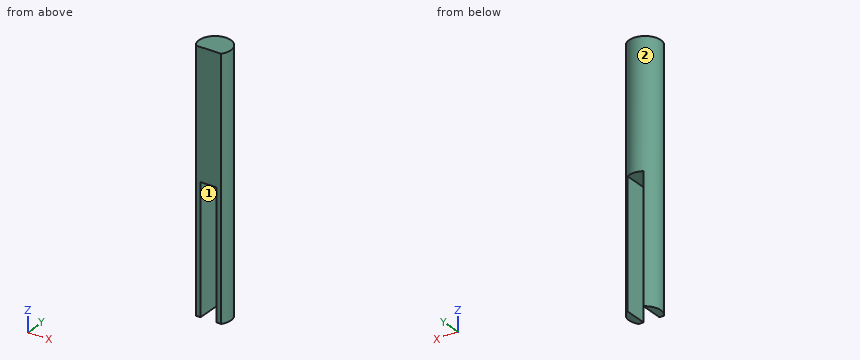
from build123d import *

# Parameters (mm, degrees)
F1_DEPTH = 50.8
F2_DEPTH = 50.8


with BuildPart() as f1:
    # F0 (on Top) → F1 (new body)
    with BuildSketch(Plane.XY):
        with BuildLine():
            Line((-3.175, -3.81), (-3.175, 5.499261314))
            ThreePointArc((-3.175, 5.499261314), (-6.2210805173, 1.2730503512), (-5.08, -3.81))
            Line((-5.08, -3.81), (-3.175, -3.81))
        make_face()
        with BuildLine():
            Line((3.175, -3.81), (3.175, 5.499261314))
            ThreePointArc((3.175, 5.499261314), (0, 6.35), (-3.175, 5.499261314))
            Line((-3.175, 5.499261314), (-3.175, -3.81))
            Line((-3.175, -3.81), (3.175, -3.81))
        make_face()
        with BuildLine():
            Line((3.175, -3.81), (5.08, -3.81))
            ThreePointArc((5.08, -3.81), (6.2210805173, 1.2730503512), (3.175, 5.499261314))
            Line((3.175, 5.499261314), (3.175, -3.81))
        make_face()
    extrude(amount=F1_DEPTH)

    # F0 (on Top) → F2 (join)
    with BuildSketch(Plane.XY):
        with BuildLine():
            Line((3.175, -3.81), (5.08, -3.81))
            ThreePointArc((5.08, -3.81), (6.2210805173, 1.2730503512), (3.175, 5.499261314))
            Line((3.175, 5.499261314), (3.175, -3.81))
        make_face()
        with BuildLine():
            Line((-3.175, -3.81), (-3.175, 5.499261314))
            ThreePointArc((-3.175, 5.499261314), (-6.2210805173, 1.2730503512), (-5.08, -3.81))
            Line((-5.08, -3.81), (-3.175, -3.81))
        make_face()
    extrude(amount=-F2_DEPTH)


solid = f1.part
Can you work these out from the model? Positions are in its coordinate system, mm. Face numbers are marked on the shaded views. A direction names the side the tool comes from. Round coordinates to 2 decimals unless told otherwise and drop trailing zeros. Write each loop counter-clockwise with the first axis right and the second up, starting at its lowest first coordinate (ties: lowest second). Pieces come first, ordered by that corner, then holes. Notation, with made-up numbers: M 16.5,-28.75 L 20.5,-28.75 A14 cw 20.5,-8.75 Z; hole C -19.75,79.25 d2. An arc over 180 degrees is marked long. Use a Markdown table: item, result.
Item 1: I want a section at C-C (x = 0). List the corners of the cut face in (y, z) for me, and give its area (3 significant figures).
Found:
| item | result |
|---|---|
| outline | M -3.81,0 L 6.35,0 L 6.35,50.8 L -3.81,50.8 Z |
| area | 516 mm2 |
Item 2: I want a section at B-B (y = 0). List the corners of the cut face in (x, z) for me (3 decimals).
Found:
| item | result |
|---|---|
| outline | M -6.35,-50.8 L -3.175,-50.8 L -3.175,0 L 3.175,0 L 3.175,-50.8 L 6.35,-50.8 L 6.35,50.8 L -6.35,50.8 Z |
Item 3: For pin 1 Ø4.5 at (y, z) = (0.5, -22.5) entering from -X; pin 2 Ø1 at (y, z) = (4, -32.5) entering from +X, each with a flat end and sliding along its axis, tell me the tip position at first contact or that it passes through.
Found:
| item | result |
|---|---|
| pin 1 | stops at x = -6.35 |
| pin 2 | stops at x = 5.3 |
Item 4: I want a section at D-D (z = 18.5). List the corners of the cut face in (x, y) for me, and give its area (3 significant figures).
Found:
| item | result |
|---|---|
| outline | M -5.08,-3.81 L 5.08,-3.81 A6.35 ccw long Z |
| area | 109 mm2 |
Item 5: Which directions (+Z, -Z, +X, -X, +Y, -Y) give clear straight access to the entire face, cutting with the end or side of a thin tool? Please do the marked faces 1 and 2.
Found:
| item | result |
|---|---|
| face 1 | -Z, +Y, -Y |
| face 2 | +Z, -Z |
Item 6: If I drill on line 1 along X through (y, z) = (-0.25, -1.5) (3 decimals); line 2 along X through (y, z) = (4, -42) (3 decimals); line 3 along Z through (x, y) = (-2.5, -1.5), over which ranges is the centre line in solid material (lowest first)? Write a range as [from, to].
Found:
| item | result |
|---|---|
| line 1 | x = [-6.345, -3.175], [3.175, 6.345] |
| line 2 | x = [-4.932, -3.175], [3.175, 4.932] |
| line 3 | z = [0, 50.8] |
Item 7: I want a section at A-A (z = -27). List the corners of the cut face in (x, y) for me (3 decimals), and give its area (3 significant figures).
Found:
| item | result |
|---|---|
| outline | M -5.08,-3.81 L -3.175,-3.81 L -3.175,5.499 A6.35 ccw Z; M 3.175,-3.81 L 5.08,-3.81 A6.35 ccw 3.175,5.499 Z |
| area | 45.9 mm2 |
